```python
from build123d import *

# Parameters (mm, degrees)
SKETCH1_W           = 450
SKETCH1_H           = 150
BOSS_EXTRUDE1_DEPTH = 3.175
CUT_EXTRUDE1_DEPTH  = 475.352274818
SKETCH3_W           = 210
SKETCH3_H           = 130
SKETCH3_W_2         = 110
SKETCH3_H_2         = 100
CUT_EXTRUDE2_DEPTH  = 475.352274818


with BuildPart() as part:
    # Sketch1 → Boss-Extrude1 (new body)
    with BuildSketch(Plane.XY):
        with Locations((225, 75)):
            Rectangle(SKETCH1_W, SKETCH1_H)
    extrude(amount=BOSS_EXTRUDE1_DEPTH)

    # Sketch2 → Cut-Extrude1 (cut, through all)
    with BuildSketch(Plane(origin=(0, 150, 0), x_dir=(1, 0, 0), z_dir=(0, 1, 0))):
        Polygon((0, -3.175), (3.175, 0), (0, 0), align=None)
        Polygon((450, -3.175), (446.825, 0), (450, 0), align=None)
    extrude(amount=-CUT_EXTRUDE1_DEPTH, mode=Mode.SUBTRACT)

    # Sketch3 → Cut-Extrude2 (cut, through all)
    with BuildSketch(Plane.XY.offset(3.175)):
        with Locations((295, 65)):
            Rectangle(SKETCH3_W, SKETCH3_H)
        with Locations((95, 75)):
            Rectangle(SKETCH3_W_2, SKETCH3_H_2)
    extrude(amount=-CUT_EXTRUDE2_DEPTH, mode=Mode.SUBTRACT)


solid = part.part
```
Here's how the part is built. I have some questions about the finished solid (model axes, mm). Coordinates: 2 decimals unless noted, no trailing zeros. Write each loop counter-clockwise with the first axis right and the second up, starting at its lowest first coordinate (ties: lowest second). Pieces come first, ordered by that corner, then holes. Notation, with made-up numbers: (81.25, -7) - (107.25, -7) arc R12 cw to (107.25, -1) - close; hole circle Ø4 at (11.25, 44). An arc over 180 degrees is marked (long way). One line per item, written item: value.
1) Suppose I cut it at B-B on x = 61.5. Write out the boundary of the cut face in (y, z) (3 decimals).
Model answer:
outline: (0, 0) - (25, 0) - (25, 3.175) - (0, 3.175) - close; (125, 0) - (150, 0) - (150, 3.175) - (125, 3.175) - close
2) Suppose I cut it at C-C on z = 2. Write out the boundary of the cut face in (x, y) (3 decimals).
Model answer:
outline: (1.175, 0) - (190, 0) - (190, 130) - (400, 130) - (400, 0) - (448.825, 0) - (448.825, 150) - (1.175, 150) - close; hole (40, 25) - (150, 25) - (150, 125) - (40, 125) - close
3) Suppose I cut it at A-A on y = 103.5. Write out the boundary of the cut face in (x, z) (3 decimals), and give its area (3 significant figures).
Model answer:
outline: (0, 3.175) - (3.175, 0) - (40, 0) - (40, 3.175) - close; (150, 0) - (190, 0) - (190, 3.175) - (150, 3.175) - close; (400, 0) - (446.825, 0) - (450, 3.175) - (400, 3.175) - close
area: 403 mm²
4) I'm going to push flat-ended pins straight in: P1, Ø1, axis at x = 288, z = 1, coming from the -Y side; P2, Ø12, axis at x = 353.5, y = 120.5, coming from the +Z side; P3, Ø1.5, axis at y = 15.5, z = 1, coming from the -X side (3 decimals). Where does each tip first touch, or does it pass through?
Model answer:
P1: stops at y = 130
P2: passes through
P3: stops at x = 1.425
5) I need wall thicknesses on line 1 along Y through (x, z) = (138.5, 2.7); line 2 along X through (y, z) = (80.5, 1.35) (3 decimals); line 3 along X through (y, z) = (32.5, 0.85) (3 decimals). Which ranges of each line are inside material? Lowest first, please.
Model answer:
line 1: y = 0 to 25, 125 to 150
line 2: x = 1.825 to 40, 150 to 190, 400 to 448.175
line 3: x = 2.325 to 40, 150 to 190, 400 to 447.675
6) Suppose I cut it at D-D on x = 198. Write out the boundary of the cut face in (y, z) (3 decimals), and give its area (3 significant figures).
Model answer:
outline: (130, 0) - (150, 0) - (150, 3.175) - (130, 3.175) - close
area: 63.5 mm²
